Verification items for the finished model (mm, model axes). A direction names the side the tool comes from. Round coordinates to 2 decimals unless told otherwise and drop trailing zeros. Loops run counter-clockwise (first coordinate to the right, second up) from the corner with the lowest first, then second, coordinate; pieces in that order, holes last. Notation, with made-up numbers: (15.5, 58) - (70.5, 58) arc R33 cw to (70.5, 86) - close; hole circle Ø2 at (66, 18.25). An arc over 180 degrees is marked (long way). Use CSV: the item, a comma, the result in double quotes.
```python
from build123d import *

# Parameters (mm, degrees)
BOSS_EXTRUDE1_DEPTH = 1.25
BOSS_EXTRUDE2_DEPTH = 2.5
BOSS_EXTRUDE2_TAPER = 25
SKETCH3_R           = 2.5
CUT_EXTRUDE1_DEPTH  = 90.193531509


with BuildPart() as part:
    # Sketch1 → Boss-Extrude1 (new, symmetric)
    with BuildSketch(Plane.XY):
        with BuildLine():
            Line((-46.61798004, 57.010347284), (-46.61798004, 48.010347284))
            ThreePointArc((-46.61798004, 48.010347284), (-42.61798004, 44.010347284), (-38.61798004, 48.010347284))
            ThreePointArc((-38.61798004, 48.010347284), (-36.630320397, 50.834381101), (-33.301202039, 49.916269553))
            ThreePointArc((-33.301202039, 49.916269553), (-22.394136584, 43.564927748), (-10.5, 47.787857357))
            ThreePointArc((-10.5, 47.787857357), (0, 52.075714714), (10.5, 47.787857357))
            ThreePointArc((10.5, 47.787857357), (22.394136584, 43.564927748), (33.301202039, 49.916269553))
            ThreePointArc((33.301202039, 49.916269553), (36.630320397, 50.834381101), (38.61798004, 48.010347284))
            ThreePointArc((38.61798004, 48.010347284), (42.61798004, 44.010347284), (46.61798004, 48.010347284))
            Line((46.61798004, 48.010347284), (46.61798004, 57.010347284))
            ThreePointArc((46.61798004, 57.010347284), (45.951330154, 59.759051808), (44.099521187, 61.89694848))
            ThreePointArc((44.099521187, 61.89694848), (0, 76), (-44.099521187, 61.89694848))
            ThreePointArc((-44.099521187, 61.89694848), (-45.951330154, 59.759051808), (-46.61798004, 57.010347284))
        make_face()
    extrude(amount=BOSS_EXTRUDE1_DEPTH, both=True)

    # Sketch2 → Boss-Extrude2 (add)
    with BuildSketch(Plane.XY.offset(1.25)):
        with BuildLine():
            ThreePointArc((24.718185374, 68.857802113), (0, 73.16), (-24.718185374, 68.857802113))
            ThreePointArc((-24.718185374, 68.857802113), (-30.323870792, 52.65411251), (-13.296533646, 50.64089234))
            ThreePointArc((-13.296533646, 50.64089234), (0, 56.07076278), (13.296533646, 50.64089234))
            ThreePointArc((13.296533646, 50.64089234), (30.323870792, 52.65411251), (24.718185374, 68.857802113))
        make_face()
    extrude(amount=BOSS_EXTRUDE2_DEPTH, taper=BOSS_EXTRUDE2_TAPER)

    # Sketch3 → Cut-Extrude1 (cut, through all)
    with BuildSketch(Plane.XY.offset(1.25)):
        with Locations((-42.61798004, 48.010347284)):
            Circle(SKETCH3_R)
        with Locations((42.61798004, 48.010347284)):
            Circle(SKETCH3_R)
    extrude(amount=-CUT_EXTRUDE1_DEPTH, mode=Mode.SUBTRACT)


solid = part.part
```
1) Cross-section at B-B, the plane y = 58.5. Record the cut outline in (x, z).
Returned:
outline,"(-46.43, -1.25) - (46.43, -1.25) - (46.43, 1.25) - (32, 1.25) - (30.84, 3.75) - (-30.84, 3.75) - (-32, 1.25) - (-46.43, 1.25) - close"
2) Thickness scan on probe 1 along X at (y, z) = (46, 0.1); probe 2 along Z at (x, y) = (-1.5, 55.5); probe 3 along X at (y, z) = (49, 2.15). Record the ranges inside material, lowest first. Write a range as [from, to].
Returned:
probe 1,"x = [-46.08, -44.1], [-41.13, -39.16], [-29.29, -12.71], [12.71, 29.29], [39.16, 41.13], [44.1, 46.08]"
probe 2,"z = [-1.25, 1.25]"
probe 3,"x = [-25.67, -16.33], [16.33, 25.67]"
3) Gauge pin test, flat ends, axial feed: pin 1 Ø10 at (x, y) = (6.5, 47) entering from +Z; pin 2 Ø1.5 at (x, z) = (-32.5, -0.5) entering from +Y; pin 3 Ø10 at (x, y) = (-30, 70.5) entering from +Z. Record the tip position at first contact, or that the pin passes through.
Returned:
pin 1,"stops at z = 1.25"
pin 2,"stops at y = 69.05"
pin 3,"stops at z = 3.41"
4) Mould release check, pull along X, two halves, no side actions. Record for faces 1 (the face through (42.53, 44.01, 0.02)), 2 (the face through (-1, 60, -1.25)), 3 (the face through (-46.618, 53, 0)): +X half, -X half, draft (parallel to the pull), parting line (faces both ways), or undercut.
Returned:
face 1,"undercut"
face 2,"draft"
face 3,"-X half"
5) Access from +Z, -Z, +X, -X, +Y, -Y to the whole of each face (thin tool, end or side, straight path). Record for faces 4 (the face through (-36.679, 50.817, 0.018)), 5 (the face through (0, 55, 1.25)).
Returned:
face 4,"+Z, -Z, -Y"
face 5,"+Z"
6) Cross-section at A-A, the plane z = 0. Record the cut outline in (x, y), then the cut area to 3 significant figures.
Returned:
outline,"(-46.62, 48.01) arc R4 ccw to (-38.62, 48.01) arc R3 cw to (-33.3, 49.92) arc R15 ccw to (-10.5, 47.79) arc R15 cw to (10.5, 47.79) arc R15 ccw to (33.3, 49.92) arc R3 cw to (38.62, 48.01) arc R4 ccw to (46.62, 48.01) - (46.62, 57.01) arc R6 ccw to (44.1, 61.9) arc R76 ccw to (-44.1, 61.9) arc R6 ccw to (-46.62, 57.01) - close; hole circle Ø5 at (-42.62, 48.01); hole circle Ø5 at (42.62, 48.01)"
area,"2,190 mm²"
